Verification items for the finished model (mm, model axes). Coordinates: 2 decimals unless noted, no trailing zeros. Write each loop counter-clockwise with the first axis right and the second up, starting at its lowest first coordinate (ties: lowest second). Pieces come first, ordered by that corner, then holes. Notation, with made-up numbers: (49.25, 7) -> (82.25, 7) arc R23 cw to (82.25, 36) -> close; hole circle Ø7 at (-30.75, -39.5). An arc over 180 degrees is marked (long way). Answer in a Markdown table with one row per item.
```python
from build123d import *

# Parameters (mm, degrees)
SKETCH2_R           = 1.75
SKETCH2_R_2         = 8
SKETCH2_R_3         = 1.7
SKETCH2_R_4         = 6
BOSS_EXTRUDE1_DEPTH = 4
FILLET1_R           = 0.5


with BuildPart() as part:
    # Sketch2 → Boss-Extrude1 (new body)
    with BuildSketch(Plane(origin=(0, 0, 0), x_dir=(1, 0, 0), z_dir=(0, 1, 0))):
        with BuildLine():
            Line((87, -11), (87, 88))
            ThreePointArc((87, 88), (84.656854249, 93.656854249), (79, 96))
            Line((79, 96), (-79, 96))
            ThreePointArc((-79, 96), (-84.656854249, 93.656854249), (-87, 88))
            Line((-87, 88), (-87, -11))
            ThreePointArc((-87, -11), (-84.656854249, -16.656854249), (-79, -19))
            Line((-79, -19), (79, -19))
            ThreePointArc((79, -19), (84.656854249, -16.656854249), (87, -11))
        make_face()
        with Locations(Location((-79, 88, 0), (0, 0, 270))):
            Circle(SKETCH2_R, mode=Mode.SUBTRACT)
        with Locations(Location((79, 88, 0), (0, 0, 270))):
            Circle(SKETCH2_R, mode=Mode.SUBTRACT)
        with Locations(Location((79, -11, 0), (0, 0, 270))):
            Circle(SKETCH2_R, mode=Mode.SUBTRACT)
        with Locations(Location((-79, -11, 0), (0, 0, 270))):
            Circle(SKETCH2_R, mode=Mode.SUBTRACT)
        with Locations(Location((0, -3, 0), (0, 0, 270))):
            Circle(SKETCH2_R_2, mode=Mode.SUBTRACT)
        with Locations(Location((18, -10.75, 0), (0, 0, 270))):
            Circle(SKETCH2_R_3, mode=Mode.SUBTRACT)
        with Locations(Location((18, 10.25, 0), (0, 0, 270))):
            Circle(SKETCH2_R_3, mode=Mode.SUBTRACT)
        with Locations(Location((-18, -10.75, 0), (0, 0, 270))):
            Circle(SKETCH2_R_3, mode=Mode.SUBTRACT)
        with Locations(Location((-18, 10.25, 0), (0, 0, 270))):
            Circle(SKETCH2_R_3, mode=Mode.SUBTRACT)
        with Locations(Location((0, 33.35, 0), (0, 0, 270))):
            Circle(SKETCH2_R_3, mode=Mode.SUBTRACT)
        with Locations(Location((18, 60.25, 0), (0, 0, 270))):
            Circle(SKETCH2_R_3, mode=Mode.SUBTRACT)
        with Locations(Location((18, 44.25, 0), (0, 0, 270))):
            Circle(SKETCH2_R_3, mode=Mode.SUBTRACT)
        with Locations(Location((-18, 44.25, 0), (0, 0, 270))):
            Circle(SKETCH2_R_3, mode=Mode.SUBTRACT)
        with Locations(Location((0, 55, 0), (0, 0, 270))):
            Circle(SKETCH2_R_4, mode=Mode.SUBTRACT)
        with Locations(Location((-18, 60.25, 0), (0, 0, 270))):
            Circle(SKETCH2_R_3, mode=Mode.SUBTRACT)
    extrude(amount=BOSS_EXTRUDE1_DEPTH)

    # Fillet1
    fillet1_edges = [part.edges().sort_by_distance(p)[0] for p in [
        (84.656854249, 4, -93.656854249),
        (0, 4, -96),
        (-84.656854249, 4, -93.656854249),
        (-87, 4, -38.5),
        (-84.656854249, 4, 16.656854249),
        (0, 4, 19),
        (84.656854249, 4, 16.656854249),
        (87, 4, -38.5),
    ]]
    fillet(fillet1_edges, radius=FILLET1_R)


solid = part.part
```
1. Material ranges on probe 1 along Z at (x, y) = (-79, 1.15); probe 2 along X at (y, z) = (3.1, -44.25); probe 3 along Z at (x, y) = (-17.5, 1.55), recorded low to high. Write a range as from..to.
Findings below:
| item | result |
|---|---|
| probe 1 | z = -96..-89.75, -86.25..9.25, 12.75..19 |
| probe 2 | x = -87..-19.7, -16.3..16.3, 19.7..87 |
| probe 3 | z = -96..-61.87, -58.63..-45.87, -42.63..-11.87, -8.63..9.13, 12.37..19 |
2. Sectioned sample at C-C, the plane z = -55. Record the cut outline in (x, y), and give its area (3 significant figures).
Findings below:
| item | result |
|---|---|
| outline | (-87, 0) -> (-6, 0) -> (-6, 4) -> (-86.5, 4) arc R0.5 ccw to (-87, 3.5) -> close; (6, 0) -> (87, 0) -> (87, 3.5) arc R0.5 ccw to (86.5, 4) -> (6, 4) -> close |
| area | 648 mm² |
3. Release check for a two-part mould opening along X. For faces 1 (the face through (-80.71, 1.97, -88.38)), 2 (the face through (-87, 2, -39)), 3 (the face through (-1, 2, 19)) record: released by +X, released by -X, zero draft, split by the parting line, or undercut.
Findings below:
| item | result |
|---|---|
| face 1 | undercut |
| face 2 | released by -X |
| face 3 | zero draft |
4. Sectioned sample at B-B, the plane z = -10.25. Record the cut outline in (x, y), and give its area (3 significant figures).
Findings below:
| item | result |
|---|---|
| outline | (-87, 0) -> (-19.7, 0) -> (-19.7, 4) -> (-86.5, 4) arc R0.5 ccw to (-87, 3.5) -> close; (-16.3, 0) -> (16.3, 0) -> (16.3, 4) -> (-16.3, 4) -> close; (19.7, 0) -> (87, 0) -> (87, 3.5) arc R0.5 ccw to (86.5, 4) -> (19.7, 4) -> close |
| area | 669 mm² |
5. Go/stop test with a flat-tipped pin: pin 1 (4.5 mm diameter, centred on x = -18, z = -60.25, fed in from +Y). Record where the tip stops, or that it passes through.
Findings below:
| item | result |
|---|---|
| pin 1 | stops at y = 4 |
6. Sectioned sample at A-A, the plane y = 1.05. Count the separate pieces of the cut face and the enclosed holes in it, and give its area (3 significant figures).
Findings below:
| item | result |
|---|---|
| separate pieces | 1 |
| enclosed holes | 15 |
| area | 19,500 mm² |
